Verification items for this drawing (mm, ordinates from the low corner). A direction names the side the tool comes from. Coordinates: 2 decimals unless noted, no trailing zeros. Order: outer loops, then holes, each group sorted by start corner. A loop starts at its lowest first (then second) coordinate and runs counter-clockwise, first axis right, second up. Notation, with made-up numbers: (68, -3) -> (99, -3) arc R17 ccw to (99, 9) -> close; hole circle Ø2 at (-8, 39.5). An arc over 180 degrees is marked (long way). Write item = value, one per line. Start each with the question number.
1. Cross-section at D-D on x = 1.5. Record the cut outline in (y, z), plus the area to 3 significant figures.
2. Cross-section at B-B on z = 11. Record the cut outline in (x, y).
3. Cross-section at A-A on x = 13. Record the cut outline in (y, z), plus the area to 3 significant figures.
4. Cross-section at C-C on y = 3.75. Record the cut outline in (x, z), plus the area to 3 significant figures.
5. Set-up check for the marked faces 1 and 2: record each of +Z, -Z, +X, -X, +Y, -Y from which the full face is reachable in a straight line by a thin tool's end or side.
6. Go/stop test with flat-tipped pins: P1, Ø0.8, axis at x = 0.5, y = 7.5, coming from the +Z side; P2, Ø3.5, axis at x = 13, z = 11, coming from the -Y side; P3, Ø0.8, axis at x = 1, y = 7.5, coming from the -Z side; P4, Ø4, axis at y = 6, z = 3, coming from the -X side. Record where each tip stops, or that it passes through.
7. Thickness scan on line 1 along Z through (x, y) = (13, 5.25); line 2 along Y through (x, z) = (13, 15.5); line 3 along X through (y, z) = (2, 9.25). Record the ranges inside material, lowest first. Write a range as from..to.
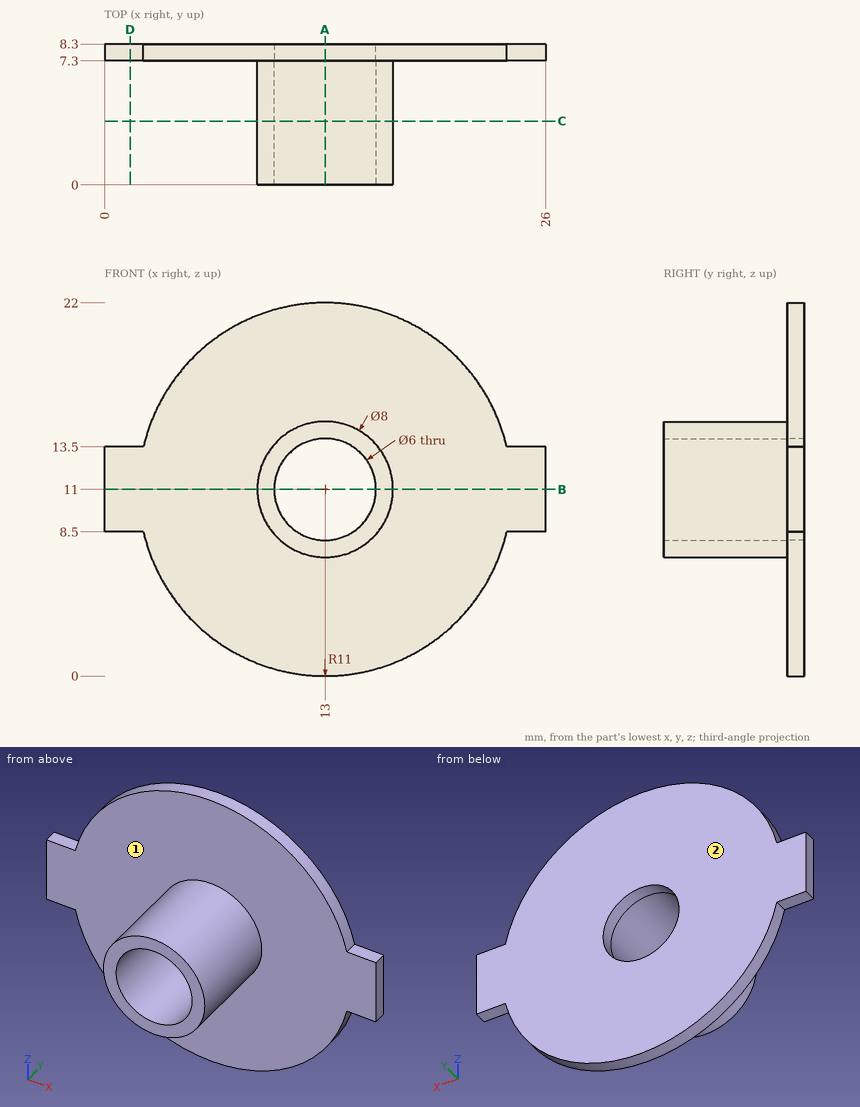
Worked out:
q1.outline = (7.3, 8.5) -> (8.3, 8.5) -> (8.3, 13.5) -> (7.3, 13.5) -> close
q1.area = 5.00 mm²
q2.outline = (0, 7.3) -> (9, 7.3) -> (9, 0) -> (10, 0) -> (10, 8.3) -> (0, 8.3) -> close; (16, 0) -> (17, 0) -> (17, 7.3) -> (26, 7.3) -> (26, 8.3) -> (16, 8.3) -> close
q3.outline = (0, 7) -> (7.3, 7) -> (7.3, 0) -> (8.3, 0) -> (8.3, 8) -> (0, 8) -> close; (0, 14) -> (8.3, 14) -> (8.3, 22) -> (7.3, 22) -> (7.3, 15) -> (0, 15) -> close
q3.area = 30.6 mm²
q4.outline = circle Ø8 at (13, 11); hole circle Ø6 at (13, 11)
q4.area = 22.0 mm²
q5.face_1 = -Y
q5.face_2 = +Z, -Z, +X, -X, +Y
q6.P1 = 13.5
q6.P2 = through
q6.P3 = 8.5
q6.P4 = 4.11
q7.line_1 = 7..8, 14..15
q7.line_2 = 7.3..8.3
q7.line_3 = 9.4..10.56, 15.44..16.6
